For this review, take the finished solid that the model builds, in its own axes (mm). Face numbers are marked on the shaded views. A direction names the side the tool comes from. Round coordinates to 2 decimals unless told otherwise and drop trailing zeros. Order: outer loops, then holes, each group sorted by start corner. A loop starts at its lowest first (then second) coordinate and runs counter-clockwise, first axis right, second up. Notation, with made-up numbers: (0, -5) - (10, -5) arc R16 ccw to (10, 22) - close; hole circle Ø3 at (-2, 28). An arc over 180 degrees is marked (long way). One line per item, written item: value.
```python
from build123d import *

# Parameters (mm, degrees)
SKETCH1_R               = 9.5
SKETCH1_R_2             = 1.7
BOSS_EXTRUDE1_DEPTH     = 9.525
SKETCH2_R               = 3.25
CUT_EXTRUDE1_DEPTH      = 5.5
SKETCH3_R               = 1.2195
CUT_EXTRUDE2_DEPTH      = 61.390194775
CUT_EXTRUDE3_REACH      = 64.926
CUT_EXTRUDE3_END_RADIUS = 9.5
SKETCH4_R               = 1.2195
CHAMFER1_SIZE           = 0.5


with BuildPart() as part:
    # Sketch1 → Boss-Extrude1 (new body)
    with BuildSketch(Plane(origin=(0, 0, 0), x_dir=(-1, 0, 0), z_dir=(0, 0, 1))):
        Polygon((-37, 0), (-37, -14), (-32.5, -14), (-32.5, -50), (-4.5, -50), (-4.5, -14), (0, -14), (0, 0), align=None)
        with Locations((-18.5, -35)):
            Circle(SKETCH1_R, mode=Mode.SUBTRACT)
        with Locations((-32.5, -7)):
            Circle(SKETCH1_R_2, mode=Mode.SUBTRACT)
        with Locations((-4.5, -7)):
            Circle(SKETCH1_R_2, mode=Mode.SUBTRACT)
    extrude(amount=BOSS_EXTRUDE1_DEPTH)

    # Sketch2 → Cut-Extrude1 (cut)
    with BuildSketch(Plane(origin=(0, 0, 0), x_dir=(-1, 0, 0), z_dir=(0, 0, -1))):
        with Locations((-32.5, 7)):
            Circle(SKETCH2_R)
        with Locations((-4.5, 7)):
            Circle(SKETCH2_R)
    extrude(amount=-CUT_EXTRUDE1_DEPTH, mode=Mode.SUBTRACT)

    # Sketch3 → Cut-Extrude2 (cut, through all)
    with BuildSketch(Plane.ZY.offset(-4.5)):
        with Locations(Location((4.7625, 35, 0), (0, 0, 270))):
            Circle(SKETCH3_R)
    extrude(amount=-CUT_EXTRUDE2_DEPTH, mode=Mode.SUBTRACT)

    # Cut-Extrude3: up to this cylinder (the profile starts outside it)
    cut_extrude3_end = Plane(origin=(18.5, 35, 4.7625), z_dir=(0, 0, -1)) * Cylinder(CUT_EXTRUDE3_END_RADIUS, 149.852, mode=Mode.PRIVATE)
    # Sketch4 → Cut-Extrude3 (cut, up to the surface)
    with BuildSketch(Plane(origin=(0, 50, 0), x_dir=(1, 0, 0), z_dir=(0, 1, 0)), mode=Mode.PRIVATE) as cut_extrude3_sk1:
        with Locations(Location((18.5, -4.7625, 0), (0, 0, 270))):
            Circle(SKETCH4_R)
    cut_extrude3_tool1 = extrude(cut_extrude3_sk1.sketch, amount=-CUT_EXTRUDE3_REACH, mode=Mode.PRIVATE) - cut_extrude3_end
    add(cut_extrude3_tool1.solids().sort_by_distance((18.5, 50, 4.7625))[0], mode=Mode.SUBTRACT)

    # Chamfer1
    chamfer1_edges = [part.edges().sort_by_distance(p)[0] for p in [
        (18.5, 50, 0),
        (32.5, 32, 0),
        (34.75, 14, 0),
        (37, 7, 0),
        (18.5, 0, 0),
        (0, 7, 0),
        (2.25, 14, 0),
        (4.5, 32, 0),
        (4.5, 32, 9.525),
        (4.5, 50, 4.7625),
        (32.5, 50, 4.7625),
        (32.5, 14, 4.7625),
        (37, 14, 4.7625),
        (37, 0, 4.7625),
        (0, 0, 4.7625),
        (0, 14, 4.7625),
        (4.5, 14, 4.7625),
        (2.25, 14, 9.525),
        (0, 7, 9.525),
        (18.5, 0, 9.525),
        (37, 7, 9.525),
        (35.75, 7, 0),
        (34.75, 14, 9.525),
        (7.75, 7, 0),
        (32.5, 32, 9.525),
        (18.5, 50, 9.525),
    ]]
    chamfer(chamfer1_edges, length=CHAMFER1_SIZE)


solid = part.part
```
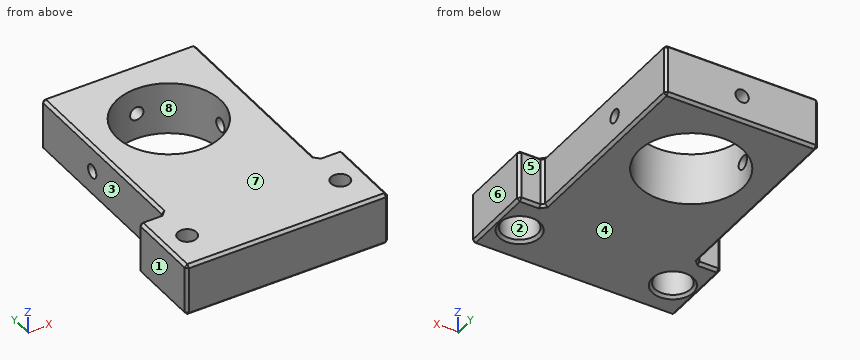
Item 1: Take a section at D-D (y = 7). Write out the cut boundary in (x, z) (3 decimals).
Returned:
outline: (0, 0.5) - (0.5, 0) - (0.75, 0) - (1.25, 0.5) - (1.25, 5.5) - (2.8, 5.5) - (2.8, 9.525) - (0.5, 9.525) - (0, 9.025) - close; (6.2, 5.5) - (7.75, 5.5) - (7.75, 0.5) - (8.25, 0) - (28.75, 0) - (29.25, 0.5) - (29.25, 5.5) - (30.8, 5.5) - (30.8, 9.525) - (6.2, 9.525) - close; (34.2, 5.5) - (35.75, 5.5) - (35.75, 0.5) - (36.25, 0) - (36.5, 0) - (37, 0.5) - (37, 9.025) - (36.5, 9.525) - (34.2, 9.525) - close
Item 2: Wall thickness on line 1 (Z direction, x = 18.5, y = 48.1) (3 decimals); line 2 (Y direction, x = 18.5, z = 2.75); line 3 (X direction, y = 8, z = 5.75): over which ranges is each line inside the solid? List them lowest first.
Returned:
line 1: 0 to 3.543, 5.982 to 9.525
line 2: 0 to 25.5, 44.5 to 50
line 3: 0 to 3.13, 5.87 to 31.13, 33.87 to 37
Item 3: Take a section at A-A (y = 35). Write out the cut boundary in (x, z) (3 decimals).
Returned:
outline: (4.5, 0.5) - (5, 0) - (9, 0) - (9, 3.543) - (4.5, 3.543) - close; (4.5, 5.982) - (9, 5.982) - (9, 9.525) - (5, 9.525) - (4.5, 9.025) - close; (28, 0) - (32, 0) - (32.5, 0.5) - (32.5, 3.543) - (28, 3.543) - close; (28, 5.982) - (32.5, 5.982) - (32.5, 9.025) - (32, 9.525) - (28, 9.525) - close
Item 4: For P1, Ø1.5, axis at y = 35, z = 4.76, coming from the -X side; P2, Ø4.5, axis at y = 36.5, z = 6.5, coming from the +X side; P3, Ø5, axis at y = 31, z = 1.5, coming from the -X side; P4, Ø5, axis at x = 32.5, y = 7, coming from the -Z side, all flat-tipped, find the tip position at first contact; note any pin that passes through.
Returned:
P1: through
P2: x = 32.5
P3: x = 4.5
P4: z = 5.5
Item 5: The part is to be moulded in two halves that separate along X. For the marked faces 6, 7 and 8, say which applies: +X half, -X half, draft (parallel to the pull), parting line (faces both ways), or undercut.
Returned:
face 6: +X half
face 7: draft
face 8: undercut
Item 6: Take a section at B-B (z = 8.25). Write out the cut boundary in (x, y), plus the area to 3 significant figures.
Returned:
outline: (0, 0.5) - (0.5, 0) - (36.5, 0) - (37, 0.5) - (37, 13.5) - (36.5, 14) - (33, 14) - (32.5, 14.5) - (32.5, 49.5) - (32, 50) - (5, 50) - (4.5, 49.5) - (4.5, 14.5) - (4, 14) - (0.5, 14) - (0, 13.5) - close; hole circle Ø3.4 at (4.5, 7); hole circle Ø19 at (18.5, 35); hole circle Ø3.4 at (32.5, 7)
area: 1,220 mm^2
Item 7: Take a section at C-C (x = 18.5). Write out the cut boundary in (y, z) (3 decimals), plus the area to 3 significant figures.
Returned:
outline: (0, 0.5) - (0.5, 0) - (25.5, 0) - (25.5, 9.525) - (0.5, 9.525) - (0, 9.025) - close; (44.5, 0) - (49.5, 0) - (50, 0.5) - (50, 3.543) - (44.5, 3.543) - close; (44.5, 5.982) - (50, 5.982) - (50, 9.025) - (49.5, 9.525) - (44.5, 9.525) - close
area: 281 mm^2
Item 8: Machinability: for the marked faces 1, 2, 3, 4 and 5, which of the approach directions +Z, -Z, +X, -X, +Y, -Y give a long, thin tool a straight path to every point of the face, cutting with its end or side? Answer none if there is none.
Returned:
face 1: +Z, -Z, -X, +Y, -Y
face 2: -Z
face 3: +Z, -Z, -X, +Y
face 4: -Z, +X, -X, +Y, -Y
face 5: +Z, -Z, +X, +Y
